```python
from build123d import *

# Parameters (mm, degrees)
F3_DEPTH  = 50.8
F5_DEPTH  = 25.4
F7_DEPTH  = 5
F8_W      = 15.135864
F8_H      = 17.9375
F9_DEPTH  = 5
F10_W     = 12.7
F10_H     = 3.2385
F11_DEPTH = 2
F13_DEPTH = 25.4


with BuildPart() as f1:
    # F0 (on Front) → F1 (revolve)
    with BuildSketch(Plane.XZ):
        with BuildLine():
            Line((0, 5), (0, 0))
            Line((0, 0), (41.7, 0))
            Line((41.7, 0), (41.7, 10.163587))
            add(Edge.make_bspline(
                [(7.75, 18.455775), (15.354575, 12.432687), (28.510841, 9.94407), (41.7, 10.163587)],
                knots=[0, 0, 0, 0, 34.948003, 34.948003, 34.948003, 34.948003], degree=3))
            Line((7.75, 18.455775), (7.75, 15.955775))
            add(Edge.make_bspline(
                [(7.75, 15.955775), (8.670718, 15.370223), (9.53974, 14.818877), (10.4, 14.3)],
                knots=[0, 0, 0, 0, 4.090011, 4.090011, 4.090011, 4.090011], degree=3))
            add(Edge.make_bspline(
                [(10.4, 14.3), (13.56972, 12.388142), (16.620486, 10.917097), (21.7, 9.8)],
                knots=[4.090011, 4.090011, 4.090011, 4.090011, 19.160091, 19.160091, 19.160091, 19.160091], degree=3))
            add(Edge.make_bspline(
                [(21.7, 9.8), (25.370522, 8.992771), (30.100394, 8.370363), (36.7, 7.9)],
                knots=[19.160091, 19.160091, 19.160091, 19.160091, 30.049925, 30.049925, 30.049925, 30.049925], degree=3))
            Line((36.7, 7.9), (36.7, 5))
            Line((36.7, 5), (21.7, 5))
            Line((21.7, 5), (10.4, 5))
            Line((10.4, 5), (0, 5))
        make_face()
    revolve(axis=Axis((0, 0, 2.5), (0, 0, -1)))

    # F2 (on Front) → F3 (cut, symmetric)
    with BuildSketch(Plane.XZ):
        Polygon((0, 5), (0, 50.867478), (-90.82243, 44.18689), (-90.82243, 5), align=None)
    extrude(amount=F3_DEPTH, both=True, mode=Mode.SUBTRACT)

    # F4 (on Top) → F5 (cut)
    with BuildSketch(Plane.XY):
        Polygon((0, -4.69055), (0, 4.69055), (-12.84133, 12.104495), (-12.84133, -12.104495), align=None)
    extrude(amount=F5_DEPTH, mode=Mode.SUBTRACT)

    # F6 (on face) → F7 (join)
    with BuildSketch(Plane(origin=(0, 0, 0), x_dir=(1, 0, 0), z_dir=(0, 0, -1))):
        Polygon((0, -4.69055), (0, 4.69055), (-12.84133, 12.104495), (-12.84133, -12.104495), align=None)
    extrude(amount=-F7_DEPTH)

    # F8 (on face) → F9 (join)
    with BuildSketch(Plane(origin=(0, 0, 0), x_dir=(1, 0, 0), z_dir=(0, 0, -1))):
        with Locations((-48.292022, 0)):
            Rectangle(F8_W, F8_H)
        with Locations((48.292022, 0)):
            Rectangle(F8_W, F8_H)
    extrude(amount=-F9_DEPTH)

    # F10 (on face) → F11 (join)
    with BuildSketch(Plane(origin=(0, 0, 0), x_dir=(1, 0, 0), z_dir=(0, 0, -1))):
        with Locations((49.509954, 1.61925)):
            Rectangle(F10_W, F10_H)
        with Locations((49.509954, -1.61925)):
            Rectangle(F10_W, F10_H)
        with Locations((-49.509954, -1.61925)):
            Rectangle(F10_W, F10_H)
        with Locations((-49.509954, 1.61925)):
            Rectangle(F10_W, F10_H)
    extrude(amount=F11_DEPTH)

    # F12 (on face) → F13 (cut)
    with BuildSketch(Plane.XY.offset(5)):
        with BuildLine():
            Line((-53.282022, 0), (-43.535147, 0))
            ThreePointArc((-43.535147, 0), (-48.408585, 4.873438), (-53.282022, 0))
        make_face()
        with BuildLine():
            ThreePointArc((-53.282022, 0), (-48.408585, -4.873438), (-43.535147, 0))
            Line((-43.535147, 0), (-53.282022, 0))
        make_face()
        with BuildLine():
            Line((43.790486, 0), (53.537361, 0))
            ThreePointArc((53.537361, 0), (48.663924, 4.873438), (43.790486, 0))
        make_face()
        with BuildLine():
            ThreePointArc((43.790486, 0), (48.663924, -4.873438), (53.537361, 0))
            Line((53.537361, 0), (43.790486, 0))
        make_face()
    extrude(amount=-F13_DEPTH, mode=Mode.SUBTRACT)


solid = f1.part
```
For this review, take the finished solid that the model builds, in its own axes (mm). A direction names the side the tool comes from. Round coordinates to 2 decimals unless told otherwise and drop trailing zeros. Write each loop counter-clockwise with the first axis right and the second up, starting at its lowest first coordinate (ties: lowest second). Pieces come first, ordered by that corner, then holes. Notation, with made-up numbers: (-18.75, 63.5) - (-9.75, 63.5) arc R25 ccw to (-9.75, 95.5) - close; hole circle Ø11 at (77, -13). An arc over 180 degrees is marked (long way). Answer as a JSON object with one key per item and string values.
1. Draft analysis for pull direction Y (two halves, no side actions). For faces 1 (the face through (-48, 8.969, 2)), 2 (the face through (-55.86, 0, 2)), 3 (the face through (0, -1, 5)), 4 (the face through (7.75, 0.17, 17.19)), state which applies: +Y half, -Y half, draft (parallel to the pull), parting line (faces both ways), or undercut.
Response values:
{"face 1": "+Y half", "face 2": "draft", "face 3": "undercut", "face 4": "undercut"}
2. Tool access review of faces 5 (the face through (-48, -8.969, 2)), 6 (the face through (48, 8.969, 2)), 7 (the face through (48, -8.969, 2)), 8 (the face through (36.69, 0.81, 6.43)), 9 (the face through (0, 26, 11)): name each direction out of +Z, -Z, +X, -X, +Y, -Y from which nothing blocks a thin tool from reaching the whole face with its end or side.
Response values:
{"face 5": "+Z, -Z, -X, -Y", "face 6": "+Z, -Z, +X, +Y", "face 7": "+Z, -Z, +X, -Y", "face 8": "-X", "face 9": "+Z, -X, +Y, -Y"}
3. We need section B-B on z = 6.5. Give the boundary of the cut face in (x, y).
Response values:
{"outline": "(0, -41.7) arc R41.7 ccw to (0, 41.7) - (0, 36.7) arc R36.7 cw to (0, -36.7) - close"}
4. To check wall thickness, follow line 1 along Z through (x, y) = (-23, -21); line 2 along Z through (x, y) = (31.5, 9); line 3 along Z through (x, y) = (28, -27). State the ranges of each line that lie inside material, in increasing order.
Response values:
{"line 1": "z = 0 to 5", "line 2": "z = 0 to 5, 8.22 to 10.44", "line 3": "z = 0 to 10.16"}
5. For pin 1 Ø0.9 at (x, z) = (44.5, -1) entering from -Y; pin 2 Ø25 at (x, y) = (-24.5, 8) entering from +Z; pin 3 Ø1.5 at (x, z) = (44.5, -1) entering from +Y, all flat-tipped, find the tip position at first contact; note any pin that passes through.
Response values:
{"pin 1": "stops at y = -3.24", "pin 2": "stops at z = 5", "pin 3": "stops at y = 3.24"}
6. We need section C-C on x = -28. Give the boundary of the cut face in (y, z).
Response values:
{"outline": "(-30.9, 0) - (30.9, 0) - (30.9, 5) - (-30.9, 5) - close"}
7. We need section A-A on x = 47.5. Give the boundary of the cut face in (y, z).
Response values:
{"outline": "(-8.97, 0) - (-4.73, 0) - (-4.73, 5) - (-8.97, 5) - close; (4.73, 0) - (8.97, 0) - (8.97, 5) - (4.73, 5) - close"}
